Input: dimensioned drawing with shaded views. Units: mm. Origin: part minimum x, y, z. A direction names the side the tool comes from. Round coordinates to 2 decimals unless told otherwise and drop trailing zeros. Loops run counter-clockwise (first coordinate to the right, second up) from the corner with the lowest first, then second, coordinate; pieces in that order, holes last. Notation, with made-up numbers: (3.25, 67) - (27.25, 67) arc R23 ccw to (27.25, 76) - close; hole circle Ø4 at (-36, 41.5). An arc over 180 degrees is marked (long way). One line per question, with ' | ' between items. Start each with the question number.
Item 1: First-contact query: pin 1 (2.5 mm diameter, centred on x = 7, y = 50, fed in from +Z); pin 2 (3 mm diameter, centred on x = 43, y = 14.5, fed in from +Z); pin 3 (2 mm diameter, centred on x = 6.41, y = 50.38, fed in from +Z). Flat tips, straight axial feed; report the tip coordinate or a pass-through.
Item 2: Section A-A, the plane z = 13.5. Return loops of the section in (x, y).
Item 3: Material intervals for line 1 along X through (y, z) = (25.5, 13); line 2 along Y through (x, z) = (12, 20); line 3 along Z through (x, y) = (85, 19), sorted ascending.
Item 4: Section C-C, the plane x = 27.5. Return loops of the section in (y, z).
Item 5: Draft query along Y for the marked faces 3, 4, 5 and 6. Return one class per face: pulls with the +Y half, pulls with the -Y half, needs draft (parallel to the pull), parting line crosses it, or undercut.
Item 6: Set-up query: the marked faces 1 and 2. Return all of +Z, -Z, +X, -X, +Y, -Y with unobstructed straight access to the full face (end or side cutting, diameter ignored); none if empty.
Item 7: Section B-B, the plane y = 20. Return loops of the section in (x, z).
Item 8: Section D-D, the plane z = 5.5. Return loops of the section in (x, y).
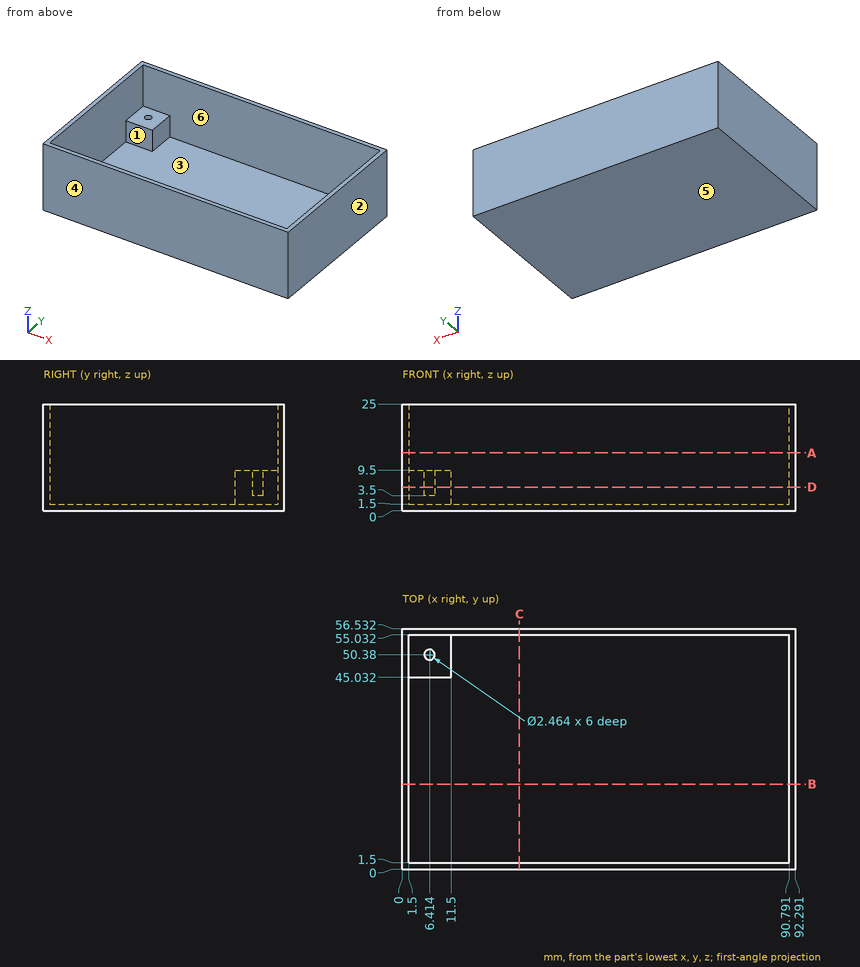
Return value:
1) pin 1: z = 9.5 | pin 2: z = 1.5 | pin 3: z = 3.5
2) outline: (0, 0) - (92.29, 0) - (92.29, 56.53) - (0, 56.53) - close; hole (1.5, 1.5) - (90.79, 1.5) - (90.79, 55.03) - (1.5, 55.03) - close
3) line 1: 0 to 1.5, 90.79 to 92.29 | line 2: 0 to 1.5, 55.03 to 56.53 | line 3: 0 to 1.5
4) outline: (0, 0) - (56.53, 0) - (56.53, 25) - (55.03, 25) - (55.03, 1.5) - (1.5, 1.5) - (1.5, 25) - (0, 25) - close
5) face 3: undercut | face 4: pulls with the -Y half | face 5: needs draft | face 6: undercut
6) face 1: +Z | face 2: +Z, -Z, +X, +Y, -Y
7) outline: (0, 0) - (92.29, 0) - (92.29, 25) - (90.79, 25) - (90.79, 1.5) - (1.5, 1.5) - (1.5, 25) - (0, 25) - close
8) outline: (0, 0) - (92.29, 0) - (92.29, 56.53) - (0, 56.53) - close; hole (1.5, 1.5) - (90.79, 1.5) - (90.79, 55.03) - (11.5, 55.03) - (11.5, 45.03) - (1.5, 45.03) - close; hole circle Ø2.46 at (6.41, 50.38)
